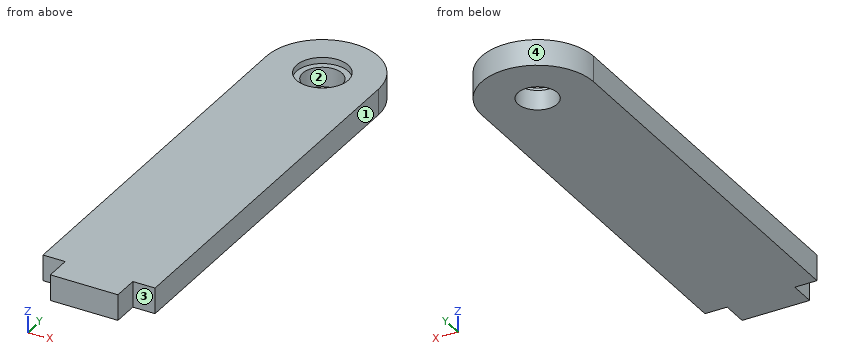
```python
from build123d import *

# Parameters (mm, degrees)
SKETCH1_R           = 4.826
SKETCH1_W           = 16.600988984
SKETCH1_H           = 6.35
BOSS_EXTRUDE1_DEPTH = 6.35
SKETCH2_R           = 6.35
SKETCH2_R_2         = 4.826
CUT_EXTRUDE1_DEPTH  = 1.524


with BuildPart() as part:
    # Sketch1 → Boss-Extrude1 (new body)
    with BuildSketch(Plane.XY):
        with BuildLine():
            Line((0, 0), (27.5, 0))
            Line((27.5, 0), (27.5, 95.25))
            ThreePointArc((27.5, 95.25), (13.75, 109), (0, 95.25))
            Line((0, 95.25), (0, 0))
        make_face()
        with Locations((13.75, 95.25)):
            Circle(SKETCH1_R, mode=Mode.SUBTRACT)
        with Locations((13.75, -3.175)):
            Rectangle(SKETCH1_W, SKETCH1_H)
    extrude(amount=BOSS_EXTRUDE1_DEPTH)

    # Sketch2 → Cut-Extrude1 (cut)
    with BuildSketch(Plane.XY.offset(6.35)):
        with Locations((13.75, 95.25)):
            Circle(SKETCH2_R)
        with Locations((13.75, 95.25)):
            Circle(SKETCH2_R_2, mode=Mode.SUBTRACT)
    extrude(amount=-CUT_EXTRUDE1_DEPTH, mode=Mode.SUBTRACT)


solid = part.part
```
Source: CAD feature listing. Evaluate the final solid. Frame: model axes, mm. Face numbers are marked on the shaded views. Coordinates: 2 decimals unless noted, no trailing zeros. Write each loop counter-clockwise with the first axis right and the second up, starting at its lowest first coordinate (ties: lowest second). Pieces come first, ordered by that corner, then holes. Notation, with made-up numbers: (63, 7.5) -> (121, 7.5) arc R14 ccw to (121, 27.5) -> close; hole circle Ø8 at (-39, 18). An arc over 180 degrees is marked (long way). Return JSON: item names as keys, results as strings. Group by question number.
1) Ray query, line 1 along Y through (x, z) = (13.75, 2.05); line 2 along Y through (x, z) = (14, 5.75); line 3 along X through (y, z) = (89.5, 5). Return the intervals inside material, ascending.
2) Contact query for flat-ended pins moving along their axis: P1, Ø3, axis at y = -3.5, z = 2, coming from the -X side; P2, Ø7.5, axis at x = 13.75, y = 95.25, coming from the -Z side. Output: stop coordinate, or through.
3) Section query B-B, the plane z = 3.75. Return loops of the section in (x, y).
4) Section query A-A, the plane x = 13.75. Return loops of the section in (y, z).
5) Mould query, pull axis Y, two halves, no side actions, for the marked faces 1, 2, 3 and 4. Classes: +Y half, -Y half, draft (parallel to the pull), parting line (faces both ways), or undercut.
From the geometry:
{
 "1": {"line 1": "-6.35 to 90.42, 100.08 to 109", "line 2": "-6.35 to 88.9, 101.6 to 109", "line 3": "0 to 11.06, 16.44 to 27.5"},
 "2": {"P1": "x = 5.45", "P2": "through"},
 "3": {"outline": "(0, 0) -> (5.45, 0) -> (5.45, -6.35) -> (22.05, -6.35) -> (22.05, 0) -> (27.5, 0) -> (27.5, 95.25) arc R13.75 ccw to (0, 95.25) -> close; hole circle Ø9.65 at (13.75, 95.25)"},
 "4": {"outline": "(-6.35, 0) -> (90.42, 0) -> (90.42, 4.83) -> (88.9, 4.83) -> (88.9, 6.35) -> (-6.35, 6.35) -> close; (100.08, 0) -> (109, 0) -> (109, 6.35) -> (101.6, 6.35) -> (101.6, 4.83) -> (100.08, 4.83) -> close"},
 "5": {"face 1": "draft", "face 2": "undercut", "face 3": "-Y half", "face 4": "+Y half"}
}
